Geometry check sheet. Reference: the model listing, model coordinates, mm. A direction names the side the tool comes from. Give positions to 0.01 mm unless a question says otherwise; leave off trailing zeros. Use a Markdown table: item, result.
```python
from build123d import *

# Parameters (mm, degrees)
SKETCH2_R          = 5
SKETCH2_R_2        = 8
CUT_EXTRUDE1_DEPTH = 20
SKETCH3_R          = 6.5
CUT_EXTRUDE2_DEPTH = 40
CUT_EXTRUDE3_START = -3
SKETCH4_R          = 122.5
CUT_EXTRUDE3_DEPTH = 3


with BuildPart() as part:
    # Sketch1 → Revolve1 (revolve)
    with BuildSketch(Plane.XY, mode=Mode.PRIVATE) as revolve1_sk:
        Polygon((0, 0), (-122.5, 0), (-122.5, 8.5), (-142, 8.5), (-142, 80), (-162.5, 80), (-162.5, 110), (-140, 110), (-140, 106), (-132, 106), (-132, 110), (-110.75, 110), (-110.75, 112.8), (-107, 112.8), (-107, 125), (-26, 125), (-26, 65), (0, 65), align=None)
    revolve(revolve1_sk.sketch.rotate(Axis((0, 0, 0), (0, 1, 0)), 270), axis=Axis((0, 0, 0), (0, 1, 0)))

    # Sketch2 → Cut-Extrude1 (cut)
    with BuildSketch(Plane.XZ):
        with Locations(Location((-111.280047836, -12.678759942, 0), (0, 0, 270))):
            Circle(SKETCH2_R)
        with Locations(Location((-111.280047836, 12.678759942, 0), (0, 0, 270))):
            Circle(SKETCH2_R)
        with Locations(Location((-105.575847002, 37.386368234, 0), (0, 0, 270))):
            Circle(SKETCH2_R)
        with Locations(Location((-94.459841931, 60.177556135, 0), (0, 0, 270))):
            Circle(SKETCH2_R)
        with Locations(Location((-105.575847002, -37.386368234, 0), (0, 0, 270))):
            Circle(SKETCH2_R)
        with Locations(Location((-94.459841931, -60.177556135, 0), (0, 0, 270))):
            Circle(SKETCH2_R)
        with Locations(Location((99.345213316, 51.715844682, 0), (0, 0, 270))):
            Circle(SKETCH2_R)
        with Locations(Location((85.165468147, 72.738181413, 0), (0, 0, 270))):
            Circle(SKETCH2_R)
        with Locations(Location((66.620152116, 90.031968389, 0), (0, 0, 270))):
            Circle(SKETCH2_R)
        with Locations(Location((44.65989572, 102.710728331, 0), (0, 0, 270))):
            Circle(SKETCH2_R)
        with Locations(Location((20.410378855, 110.124549647, 0), (0, 0, 270))):
            Circle(SKETCH2_R)
        with Locations(Location((-4.885371385, 111.893400817, 0), (0, 0, 270))):
            Circle(SKETCH2_R)
        with Locations(Location((-4.885371385, -111.893400817, 0), (0, 0, 270))):
            Circle(SKETCH2_R)
        with Locations(Location((20.410378855, -110.124549647, 0), (0, 0, 270))):
            Circle(SKETCH2_R)
        with Locations(Location((44.65989572, -102.710728331, 0), (0, 0, 270))):
            Circle(SKETCH2_R)
        with Locations(Location((66.620152116, -90.031968389, 0), (0, 0, 270))):
            Circle(SKETCH2_R)
        with Locations(Location((85.165468147, -72.738181413, 0), (0, 0, 270))):
            Circle(SKETCH2_R)
        with Locations(Location((99.345213316, -51.715844682, 0), (0, 0, 270))):
            Circle(SKETCH2_R)
        with Locations(Location((-84.693466759, 14.933743279, 0), (0, 0, 270))):
            Circle(SKETCH2_R_2)
        with Locations(Location((-84.693466759, -14.933743279, 0), (0, 0, 270))):
            Circle(SKETCH2_R_2)
        with Locations(Location((55.279734433, 65.879822108, 0), (0, 0, 270))):
            Circle(SKETCH2_R_2)
        with Locations(Location((29.413732326, 80.813565388, 0), (0, 0, 270))):
            Circle(SKETCH2_R_2)
        with Locations(Location((29.413732326, -80.813565388, 0), (0, 0, 270))):
            Circle(SKETCH2_R_2)
        with Locations(Location((55.279734433, -65.879822108, 0), (0, 0, 270))):
            Circle(SKETCH2_R_2)
    extrude(amount=-CUT_EXTRUDE1_DEPTH, mode=Mode.SUBTRACT)

    # Sketch3 → Cut-Extrude2 (cut)
    with BuildSketch(Plane.XZ.offset(-80)):
        with Locations(Location((0, 152, 0), (0, 0, 270))):
            Circle(SKETCH3_R)
        with Locations(Location((58.167881719, 140.429688942, 0), (0, 0, 270))):
            Circle(SKETCH3_R)
        with Locations(Location((107.48023074, 107.48023074, 0), (0, 0, 270))):
            Circle(SKETCH3_R)
        with Locations(Location((140.429688942, 58.167881719, 0), (0, 0, 270))):
            Circle(SKETCH3_R)
        with Locations(Location((152, 0, 0), (0, 0, 270))):
            Circle(SKETCH3_R)
        with Locations(Location((140.429688942, -58.167881719, 0), (0, 0, 270))):
            Circle(SKETCH3_R)
        with Locations(Location((107.48023074, -107.48023074, 0), (0, 0, 270))):
            Circle(SKETCH3_R)
        with Locations(Location((58.167881719, -140.429688942, 0), (0, 0, 270))):
            Circle(SKETCH3_R)
        with Locations(Location((0, -152, 0), (0, 0, 270))):
            Circle(SKETCH3_R)
        with Locations(Location((-58.167881719, -140.429688942, 0), (0, 0, 270))):
            Circle(SKETCH3_R)
        with Locations(Location((-107.48023074, -107.48023074, 0), (0, 0, 270))):
            Circle(SKETCH3_R)
        with Locations(Location((-140.429688942, -58.167881719, 0), (0, 0, 270))):
            Circle(SKETCH3_R)
        with Locations(Location((-152, 0, 0), (0, 0, 270))):
            Circle(SKETCH3_R)
        with Locations(Location((-140.429688942, 58.167881719, 0), (0, 0, 270))):
            Circle(SKETCH3_R)
        with Locations(Location((-107.48023074, 107.48023074, 0), (0, 0, 270))):
            Circle(SKETCH3_R)
        with Locations(Location((-58.167881719, 140.429688942, 0), (0, 0, 270))):
            Circle(SKETCH3_R)
    extrude(amount=-CUT_EXTRUDE2_DEPTH, mode=Mode.SUBTRACT)

    # Sketch4 → Cut-Extrude3 (cut)
    with BuildSketch(Plane.XZ.offset(CUT_EXTRUDE3_START)):
        with Locations(Location((0, 0, 0), (0, 0, 270))):
            Circle(SKETCH4_R)
        with BuildLine():
            ThreePointArc((20.232592114, 60.717725718), (-58.25, 100.891959541), (-62.699388989, 12.836924104))
            ThreePointArc((-62.699388989, 12.836924104), (-64, 0), (-62.699388989, -12.836924104))
            ThreePointArc((-62.699388989, -12.836924104), (-58.25, -100.891959541), (20.232592114, -60.717725718))
            ThreePointArc((20.232592114, -60.717725718), (32, -55.425625842), (42.466796875, -47.880801614))
            ThreePointArc((42.466796875, -47.880801614), (116.5, 0), (42.466796875, 47.880801614))
            ThreePointArc((42.466796875, 47.880801614), (32, 55.425625842), (20.232592114, 60.717725718))
        make_face(mode=Mode.SUBTRACT)
    extrude(amount=CUT_EXTRUDE3_DEPTH, mode=Mode.SUBTRACT)


solid = part.part
```
1) Depth check by flat-ended pin: P1, Ø10, axis at y = 36, z = 11, coming from the -X side; P2, Ø5, axis at x = -92.5, z = 60.5, coming from the -Y side; P3, Ø11, axis at x = -93.5, z = -61, coming from the -Y side; P4, Ø11.5, axis at x = 58.17, z = -140.43, coming from the -Y side. Enter the tip coordinate at first touch or a pass-through.
Working result:
| item | result |
|---|---|
| P1 | stops at x = -141.87 |
| P2 | stops at y = 20 |
| P3 | stops at y = 3 |
| P4 | passes through |
2) Section check A-A on z = 0. Count the separate pieces of the cut face and the enclosed holes in it, then the cut area to 3 significant figures.
Working result:
| item | result |
|---|---|
| separate pieces | 3 |
| enclosed holes | 0 |
| area | 31,200 mm² |
3) Material ranges on L1, parallel to Z at x = -81, y = 11; L2, parallel to Y at x = -7.5, z = -138; L3, parallel to Y at x = -105, z = -35, recorded low to high. Write a range as from..to.
Working result:
| item | result |
|---|---|
| L1 | z = -116.63..-22.03, -7.84..7.84, 22.03..116.63 |
| L2 | y = 8.5..106 |
| L3 | y = 20..112.8 |
4) Set-up check for faces 1 (the flat face through (-106, 20, -37)), 2 (the cylindrical face through (15.821, 94.58, 20.633)), 3 (the cylindrical face through (32.157, 1.521, 55.335)), 4 (the cylindrical face through (113.925, 94.79, -106.634)): record each of +Z, -Z, +X, -X, +Y, -Y from which the full face is reachable in a straight line by a thin tool's end or side.
Working result:
| item | result |
|---|---|
| face 1 | -Y |
| face 2 | +Y |
| face 3 | +Z, -Y |
| face 4 | +Y, -Y |
5) Mould release check, pull along X, two halves, no side actions. Record for faces 5 (the flat face through (-111, 20, 13)), 6 (the flat face through (-121, 110, 73)): pulls with the +X half, pulls with the -X half, needs draft (parallel to the pull), parting line crosses it, or undercut.
Working result:
| item | result |
|---|---|
| face 5 | undercut |
| face 6 | needs draft |
